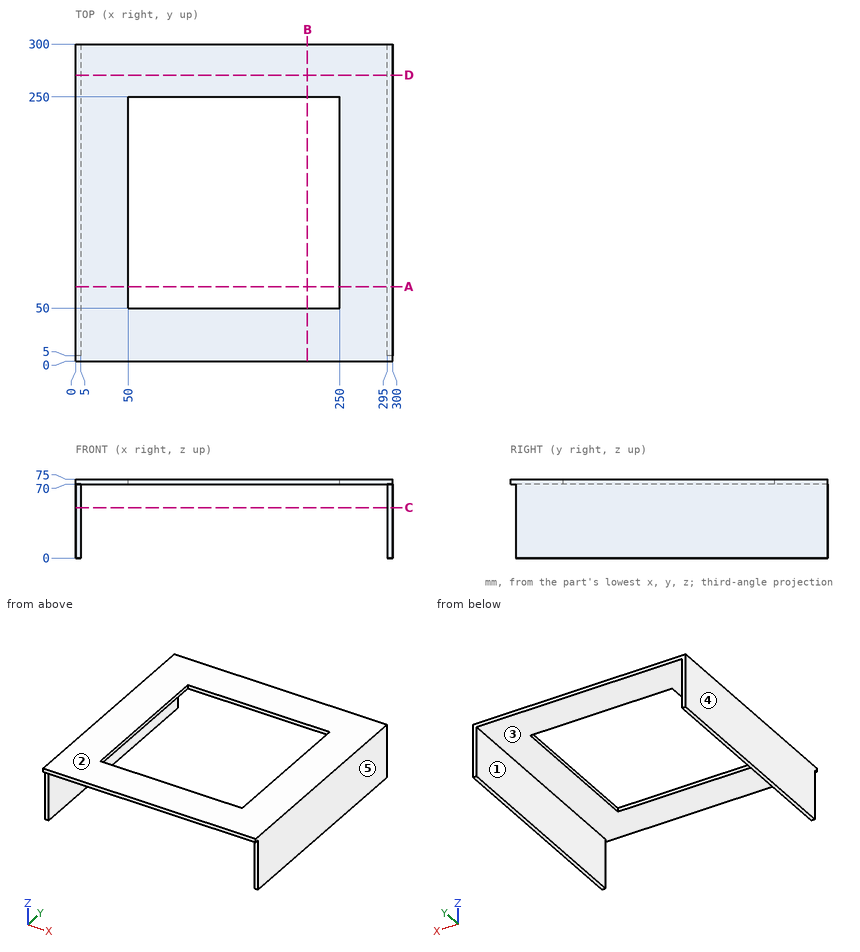
Geometry check sheet. Reference: drawing and pictorial views, mm from the part's lowest x, y, z. A direction names the side the tool comes from. Give positions to 0.01 mm unless a question says otherwise; leave off trailing zeros. Write each loop counter-clockwise with the first axis right and the second up, starting at its lowest first coordinate (ties: lowest second). Pieces come first, ordered by that corner, then holes. Notation, with made-up numbers: M -13.75,-7.75 L 36.25,-7.75 A22 ccw 36.25,0.25 Z; hole C 53,50.25 d9. An arc over 180 degrees is marked long. Put each result on its own line as item: value. Start each with the question number.
1. Section check A-A (y = 70.5). Record the cut outline in (x, z), and give its area (3 significant figures).
2. Section check C-C (z = 48). Record the cut outline in (x, y).
3. Set-up check for the marked faces 1 and 2: record each of +Z, -Z, +X, -X, +Y, -Y from which the full face is reachable in a straight line by a thin tool's end or side.
4. Section check D-D (y = 270.5). Record the cut outline in (x, z), and give its area (3 significant figures).
5. Scan lines: line 1 along X through (y, z) = (19, 3.5); line 2 along Z through (x, y) = (42, 266). Record each from-to range of solid material in increasing order. Write a range as [from, to].
6. Section check B-B (x = 219.5). Record the cut outline in (y, z), and give its area (3 significant figures).
7. Go/stop test with flat-tipped pins: pin 1 Ø3 at (x, z) = (248, 67) entering from +Y; pin 2 Ø5.5 at (x, z) = (1.5, 31) entering from -Y; pin 3 Ø5.5 at (y, z) = (110, 73) entering from -X. Record where each tip stops, or that it passes through.
8. Draft check along X on the marked faces 3, 4 and 5. Enter one of: +X half, -X half, draft (parallel to the pull), parting line (faces both ways), or undercut.
Answer list:
1. outline: M 0,0 L 5,0 L 5,70 L 50,70 L 50,75 L 0,75 Z; M 250,70 L 295,70 L 295,0 L 300,0 L 300,75 L 250,75 Z
1. area: 1,200 mm2
2. outline: M 0,5 L 5,5 L 5,300 L 0,300 Z; M 295,5 L 300,5 L 300,300 L 295,300 Z
3. face 1: -Z, +Y, -Y
3. face 2: +Z, +X, -X, +Y, -Y
4. outline: M 0,0 L 5,0 L 5,70 L 295,70 L 295,0 L 300,0 L 300,75 L 0,75 Z
4. area: 2,200 mm2
5. line 1: [0, 5], [295, 300]
5. line 2: [70, 75]
6. outline: M 0,70 L 50,70 L 50,75 L 0,75 Z; M 250,70 L 300,70 L 300,75 L 250,75 Z
6. area: 500 mm2
7. pin 1: through
7. pin 2: y = 5
7. pin 3: x = 0
8. face 3: undercut
8. face 4: -X half
8. face 5: +X half
